Geometry check sheet. Reference: the model listing, model coordinates, mm. Coordinates: 2 decimals unless noted, no trailing zeros. Loops run counter-clockwise (first coordinate to the right, second up) from the corner with the lowest first, then second, coordinate; pieces in that order, holes last.
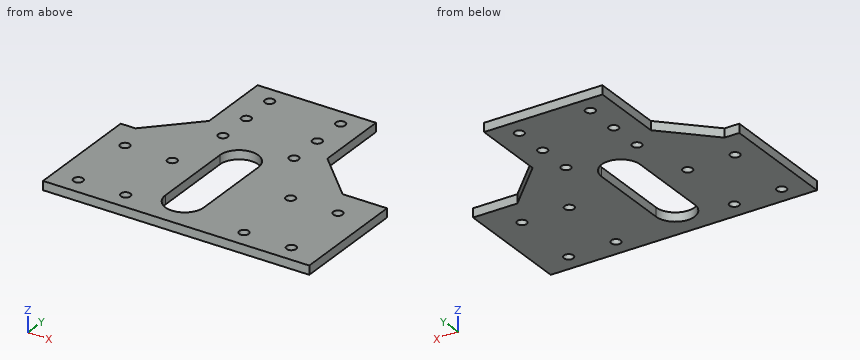
from build123d import *

# Parameters (mm, degrees)
EXTRUDE_1_DEPTH     = 3
SKETCH_2_R          = 1.6
CUT_EXTRUDE_1_DEPTH = 3


with BuildPart() as part:
    # 草图1 → 凸台-拉伸1 (new body)
    with BuildSketch(Plane.XY):
        Polygon((0, 0), (0, 40), (5, 40), (20, 55), (20, 80), (60, 80), (60, 55), (75, 40), (90, 40), (90, 0), align=None)
    extrude(amount=EXTRUDE_1_DEPTH)

    # 草图2 → 切除-拉伸1 (cut)
    with BuildSketch(Plane.XY.offset(3)):
        with Locations((28, 74)):
            Circle(SKETCH_2_R)
        with Locations((28, 50)):
            Circle(SKETCH_2_R)
        with Locations((52, 74)):
            Circle(SKETCH_2_R)
        with Locations((52, 50)):
            Circle(SKETCH_2_R)
        with Locations((8, 30)):
            Circle(SKETCH_2_R)
        with Locations((24, 30)):
            Circle(SKETCH_2_R)
        with Locations((80, 30)):
            Circle(SKETCH_2_R)
        with Locations((64, 30)):
            Circle(SKETCH_2_R)
        with Locations((80, 6)):
            Circle(SKETCH_2_R)
        with Locations((64, 6)):
            Circle(SKETCH_2_R)
        with Locations((24, 6)):
            Circle(SKETCH_2_R)
        with Locations((8, 6)):
            Circle(SKETCH_2_R)
        with Locations((28, 62)):
            Circle(SKETCH_2_R)
        with Locations((52, 62)):
            Circle(SKETCH_2_R)
        with BuildLine():
            Line((46.5, 40), (46.5, 12))
            ThreePointArc((46.5, 12), (40, 5.5), (33.5, 12))
            Line((33.5, 12), (33.5, 40))
            ThreePointArc((33.5, 40), (40, 46.5), (46.5, 40))
        make_face()
    extrude(amount=-CUT_EXTRUDE_1_DEPTH, mode=Mode.SUBTRACT)


solid = part.part
(1) Sectioned sample at D-D on x = 52. Record the cut outline in (y, z), and give its area (3 significant figures).
Findings:
outline: (0, 0) - (48.4, 0) - (48.4, 3) - (0, 3) - close; (51.6, 0) - (60.4, 0) - (60.4, 3) - (51.6, 3) - close; (63.6, 0) - (72.4, 0) - (72.4, 3) - (63.6, 3) - close; (75.6, 0) - (80, 0) - (80, 3) - (75.6, 3) - close
area: 211 mm2
(2) Gauge pin test, flat ends, axial feed: pin 1 Ø3 at (x, y) = (8, 30) entering from -Z; pin 2 Ø0.9 at (y, z) = (69, 1) entering from +X; pin 3 Ø1.5 at (x, z) = (80, 1) entering from +Y. Record the tip position at first contact, or that the pin passes through.
Findings:
pin 1: passes through
pin 2: stops at x = 60
pin 3: stops at y = 40
(3) Scan lines: L1, parallel to Y at x = 52, z = 1.45; L2, parallel to X at y = 74, z = 0.75; L3, parallel to X at y = 14, z = 1.5. Record each from-to range of solid material in increasing order.
Findings:
L1: y = 0 to 48.4, 51.6 to 60.4, 63.6 to 72.4, 75.6 to 80
L2: x = 20 to 26.4, 29.6 to 50.4, 53.6 to 60
L3: x = 0 to 33.5, 46.5 to 90
(4) Sectioned sample at C-C on z = 1.4. State how many separate pieces and enclosed holes the cut face has, and give its area (3 significant figures).
Findings:
separate pieces: 1
enclosed holes: 15
area: 4,820 mm2
(5) Sectioned sample at B-B on x = 40. Record the cut outline in (y, z), and give its area (3 significant figures).
Findings:
outline: (0, 0) - (5.5, 0) - (5.5, 3) - (0, 3) - close; (46.5, 0) - (80, 0) - (80, 3) - (46.5, 3) - close
area: 117 mm2
(6) Sectioned sample at A-A on y = 15. Record the cut outline in (x, z).
Findings:
outline: (0, 0) - (33.5, 0) - (33.5, 3) - (0, 3) - close; (46.5, 0) - (90, 0) - (90, 3) - (46.5, 3) - close
